Could you check a few things on this model? Use its own coordinates, in mm. A direction names the side the tool comes from. Give positions to 0.01 mm unless a question says otherwise; leave off trailing zeros. Order: outer loops, then holes, each group sorted by start corner. A loop starts at its lowest first (then second) coordinate and runs counter-clockwise, first axis right, second up. Notation, with made-up numbers: M 26,9.5 L 76,9.5 A20 ccw 76,40.5 Z; hole C 39,33 d11. An arc over 180 degrees is marked long. Use a Markdown table: item, result. Add a question column.
```python
from build123d import *

# Parameters (mm, degrees)
BOSS_EXTRU_1_DEPTH = 3


with BuildPart() as part:
    # Esquisse1 → Boss.-Extru.1 (new body)
    with BuildSketch(Plane.XY):
        with BuildLine():
            Line((-119.34630187, 4.320852512), (-119.346382005, -12.429484403))
            Line((-119.346382005, -12.429484403), (-101.345774335, -12.429484403))
            Line((-101.345774335, -12.429484403), (-101.345774335, -9.929307079))
            Line((-101.345774335, -9.929307079), (-82.803225752, -9.929307079))
            Line((-82.803225752, -9.929307079), (-82.803225752, -7.679926158))
            Line((-82.803225752, -7.679926158), (-62.801949021, -7.681038584))
            Line((-62.801949021, -7.681038584), (-62.801949021, -9.929307079))
            Line((-62.801949021, -9.929307079), (-43.80060136, -9.929307079))
            Line((-43.80060136, -9.929307079), (-43.80060136, -14.679643994))
            Line((-43.80060136, -14.679643994), (-5.797906039, -14.679643994))
            Line((-5.797906039, -14.679643994), (-5.797906039, -72.933633781))
            Line((-5.797906039, -72.933633781), (-61.577157206, -72.933633781))
            Line((-61.577157206, -72.933633781), (-72.263087593, -87.572177036))
            Line((-72.263087593, -87.572177036), (-109.761976756, -93.1463556))
            Line((-109.761976756, -93.1463556), (-126.111124489, -102.556497988))
            Line((-126.111124489, -102.556497988), (-140.02282508, -78.342807898))
            Line((-140.02282508, -78.342807898), (-140.02282508, 4.320852512))
            Line((-140.02282508, 4.320852512), (-142.02282508, 4.320852512))
            Line((-142.02282508, 4.320852512), (-154.65055875, 4.320852512))
            Line((-154.65055875, 4.320852512), (-158.478985875, 0.492425388))
            Line((-158.478985875, 0.492425388), (-158.478985875, -3.429484403))
            Line((-158.478985875, -3.429484403), (-158.478985875, -70.307502815))
            Line((-158.478985875, -70.307502815), (-132.440036759, -115.628996046))
            Line((-132.440036759, -115.628996046), (-127.216265437, -117.03834868))
            Line((-127.216265437, -117.03834868), (-105.747438988, -104.681452952))
            Line((-105.747438988, -104.681452952), (-65.531582138, -98.70339941))
            Line((-65.531582138, -98.70339941), (-55.479847181, -84.933633781))
            Line((-55.479847181, -84.933633781), (2.202093961, -84.933633781))
            Line((2.202093961, -84.933633781), (7.202093961, -79.933633781))
            Line((7.202093961, -79.933633781), (7.202093961, -0.684932032))
            Line((7.202093961, -0.684932032), (2.202093969, 4.315346056))
            Line((2.202093969, 4.315346056), (-5.797906039, 4.315790998))
            Line((-5.797906039, 4.315790998), (-5.797906039, -5.684153384))
            ThreePointArc((-5.797906039, -5.684153384), (-6.797906039, -6.684153384), (-7.797906039, -5.684153384))
            Line((-7.797906039, -5.684153384), (-7.797906039, 4.315902234))
            Line((-7.797906039, 4.315902234), (-9.797906039, 4.316013469))
            Line((-9.797906039, 4.316013469), (-9.797906039, -5.684153384))
            ThreePointArc((-9.797906039, -5.684153384), (-10.797906039, -6.684153384), (-11.797906039, -5.684153384))
            Line((-11.797906039, -5.684153384), (-11.797906039, 4.316124705))
            Line((-11.797906039, 4.316124705), (-13.797906039, 4.31623594))
            Line((-13.797906039, 4.31623594), (-13.797906039, -5.684153384))
            ThreePointArc((-13.797906039, -5.684153384), (-14.797906039, -6.684153384), (-15.797906039, -5.684153384))
            Line((-15.797906039, -5.684153384), (-15.797906039, 4.316347176))
            Line((-15.797906039, 4.316347176), (-17.797906039, 4.316458411))
            Line((-17.797906039, 4.316458411), (-17.797906039, -5.684153384))
            ThreePointArc((-17.797906039, -5.684153384), (-18.797906039, -6.684153384), (-19.797906039, -5.684153384))
            Line((-19.797906039, -5.684153384), (-19.797906039, 4.316569647))
            Line((-19.797906039, 4.316569647), (-21.797906039, 4.316680882))
            Line((-21.797906039, 4.316680882), (-21.797906039, -5.684153384))
            ThreePointArc((-21.797906039, -5.684153384), (-22.797906039, -6.684153384), (-23.797906039, -5.684153384))
            Line((-23.797906039, -5.684153384), (-23.797906039, 4.316792118))
            Line((-23.797906039, 4.316792118), (-25.797906039, 4.316903353))
            Line((-25.797906039, 4.316903353), (-25.797906039, -5.684153384))
            ThreePointArc((-25.797906039, -5.684153384), (-26.797906039, -6.684153384), (-27.797906039, -5.684153384))
            Line((-27.797906039, -5.684153384), (-27.797906039, 4.317014589))
            Line((-27.797906039, 4.317014589), (-29.797906039, 4.317125824))
            Line((-29.797906039, 4.317125824), (-29.797906039, -5.684153384))
            ThreePointArc((-29.797906039, -5.684153384), (-30.797906039, -6.684153384), (-31.797906039, -5.684153384))
            Line((-31.797906039, -5.684153384), (-31.797906039, 4.31723706))
            Line((-31.797906039, 4.31723706), (-33.797906039, 4.317348295))
            Line((-33.797906039, 4.317348295), (-33.797906039, -5.684153384))
            ThreePointArc((-33.797906039, -5.684153384), (-34.797906039, -6.684153384), (-35.797906039, -5.684153384))
            Line((-35.797906039, -5.684153384), (-35.797906039, 4.317459531))
            Line((-35.797906039, 4.317459531), (-37.797906039, 4.317570766))
            Line((-37.797906039, 4.317570766), (-37.797906039, -5.684153384))
            ThreePointArc((-37.797906039, -5.684153384), (-38.797906039, -6.684153384), (-39.797906039, -5.684153384))
            Line((-39.797906039, -5.684153384), (-39.797906039, 4.317682002))
            Line((-39.797906039, 4.317682002), (-41.797906039, 4.317793237))
            Line((-41.797906039, 4.317793237), (-41.797906039, -5.684153384))
            ThreePointArc((-41.797906039, -5.684153384), (-42.797906039, -6.684153384), (-43.797906039, -5.684153384))
            Line((-43.797906039, -5.684153384), (-43.797906039, 4.317904473))
            Line((-43.797906039, 4.317904473), (-45.797906039, 4.318015708))
            Line((-45.797906039, 4.318015708), (-45.797906039, -5.684153384))
            ThreePointArc((-45.797906039, -5.684153384), (-46.797906039, -6.684153384), (-47.797906039, -5.684153384))
            Line((-47.797906039, -5.684153384), (-47.797906039, 4.318126944))
            Line((-47.797906039, 4.318126944), (-49.797906039, 4.318238179))
            Line((-49.797906039, 4.318238179), (-49.797906039, -5.684153384))
            ThreePointArc((-49.797906039, -5.684153384), (-50.797906039, -6.684153384), (-51.797906039, -5.684153384))
            Line((-51.797906039, -5.684153384), (-51.797906039, 4.318349415))
            Line((-51.797906039, 4.318349415), (-53.797906039, 4.31846065))
            Line((-53.797906039, 4.31846065), (-53.797906039, -5.684153384))
            ThreePointArc((-53.797906039, -5.684153384), (-54.797906039, -6.684153384), (-55.797906039, -5.684153384))
            Line((-55.797906039, -5.684153384), (-55.797906039, 4.318571886))
            Line((-55.797906039, 4.318571886), (-57.797906039, 4.318683121))
            Line((-57.797906039, 4.318683121), (-57.797906039, -5.684153384))
            ThreePointArc((-57.797906039, -5.684153384), (-58.797906039, -6.684153384), (-59.797906039, -5.684153384))
            Line((-59.797906039, -5.684153384), (-59.797906039, 4.318794357))
            Line((-59.797906039, 4.318794357), (-61.797906039, 4.318905592))
            Line((-61.797906039, 4.318905592), (-61.797906039, -5.684153384))
            ThreePointArc((-61.797906039, -5.684153384), (-62.797906039, -6.684153384), (-63.797906039, -5.684153384))
            Line((-63.797906039, -5.684153384), (-63.797906039, 4.319016828))
            Line((-63.797906039, 4.319016828), (-65.797906039, 4.319128063))
            Line((-65.797906039, 4.319128063), (-65.797906039, -5.684153384))
            ThreePointArc((-65.797906039, -5.684153384), (-66.797906039, -6.684153384), (-67.797906039, -5.684153384))
            Line((-67.797906039, -5.684153384), (-67.797906039, 4.319239299))
            Line((-67.797906039, 4.319239299), (-69.797906039, 4.319350534))
            Line((-69.797906039, 4.319350534), (-69.797906039, -5.684153384))
            ThreePointArc((-69.797906039, -5.684153384), (-70.797906039, -6.684153384), (-71.797906039, -5.684153384))
            Line((-71.797906039, -5.684153384), (-71.797906039, 4.31946177))
            Line((-71.797906039, 4.31946177), (-73.797906039, 4.319573005))
            Line((-73.797906039, 4.319573005), (-73.797906039, -5.684153384))
            ThreePointArc((-73.797906039, -5.684153384), (-74.797906039, -6.684153384), (-75.797906039, -5.684153384))
            Line((-75.797906039, -5.684153384), (-75.797906039, 4.319684241))
            Line((-75.797906039, 4.319684241), (-77.797906039, 4.319795476))
            Line((-77.797906039, 4.319795476), (-77.797906039, -5.684153384))
            ThreePointArc((-77.797906039, -5.684153384), (-78.797906039, -6.684153384), (-79.797906039, -5.684153384))
            Line((-79.797906039, -5.684153384), (-79.797906039, 4.319906712))
            Line((-79.797906039, 4.319906712), (-81.797906039, 4.320017947))
            Line((-81.797906039, 4.320017947), (-81.797906039, -5.684153384))
            ThreePointArc((-81.797906039, -5.684153384), (-82.797906039, -6.684153384), (-83.797906039, -5.684153384))
            Line((-83.797906039, -5.684153384), (-83.797906039, 4.320129183))
            Line((-83.797906039, 4.320129183), (-85.797906039, 4.320240418))
            Line((-85.797906039, 4.320240418), (-85.797906039, -5.684153384))
            ThreePointArc((-85.797906039, -5.684153384), (-86.797906039, -6.684153384), (-87.797906039, -5.684153384))
            Line((-87.797906039, -5.684153384), (-87.797906039, 4.320351654))
            Line((-87.797906039, 4.320351654), (-89.797906039, 4.320462889))
            Line((-89.797906039, 4.320462889), (-89.797906039, -5.684153384))
            ThreePointArc((-89.797906039, -5.684153384), (-90.797906039, -6.684153384), (-91.797906039, -5.684153384))
            Line((-91.797906039, -5.684153384), (-91.797906039, 4.320574125))
            Line((-91.797906039, 4.320574125), (-93.797906039, 4.32068536))
            Line((-93.797906039, 4.32068536), (-93.797906039, -5.684153384))
            ThreePointArc((-93.797906039, -5.684153384), (-94.797906039, -6.684153384), (-95.797906039, -5.684153384))
            Line((-95.797906039, -5.684153384), (-95.797906039, 4.320796596))
            Line((-95.797906039, 4.320796596), (-96.80328137, 4.320852512))
            Line((-96.80328137, 4.320852512), (-97.797906039, 4.320852512))
            Line((-97.797906039, 4.320852512), (-97.797906039, -5.684153384))
            ThreePointArc((-97.797906039, -5.684153384), (-98.797906039, -6.684153384), (-99.797906039, -5.684153384))
            Line((-99.797906039, -5.684153384), (-99.797906039, 4.320852512))
            Line((-99.797906039, 4.320852512), (-101.797906039, 4.320852512))
            Line((-101.797906039, 4.320852512), (-101.797906039, -5.684153384))
            ThreePointArc((-101.797906039, -5.684153384), (-102.797906039, -6.684153384), (-103.797906039, -5.684153384))
            Line((-103.797906039, -5.684153384), (-103.797906039, 4.320852512))
            Line((-103.797906039, 4.320852512), (-103.799739609, 4.320852512))
            Line((-103.799739609, 4.320852512), (-117.346315028, 4.320852512))
            Line((-117.346315028, 4.320852512), (-119.34630187, 4.320852512))
        make_face()
    extrude(amount=BOSS_EXTRU_1_DEPTH)


solid = part.part
```
1) Suppose I cut it at B-B on y = -95.5. Please give me the cut outline in (x, z), and give its area (3 significant figures).
2) For faces 1 (the face through (-51, -74, 3)), 2 (the face through (-66.845, -80.15, 1.479)), 3 (the face through (-132.97, -90.62, 1.48)), which set-ups out of +Z, -Z, +X, -X, +Y, -Y let a thin tool reach every point of the face, with its end or its side?
3) Please list where these lines run through material, in increasing order: line 1 (X direction, y = -10.5, z = 1); line 2 (Y direction, x = -59, z = 2.35); line 3 (X direction, y = -69.5, z = 0.65). Write a range as from..to.
4) For pin 1 (0.9 mm diameter, centred on y = 1, z = 1.5, fed in from -X); pin 2 (1.5 mm diameter, centred on y = 0.5, z = 2, fed in from +X); pin 3 (1 mm diameter, centred on x = -48.5, z = 1, fed in from +Y), each with a flat end and sliding along its axis, tell me the tip position at first contact or that it passes through.
5) Suppose I cut it at C-C on x = -129. Please give me the cut outline in (y, z), and give its area (3 significant figures).
6) Suppose I cut it at A-A on y = -56. Please give me the cut outline in (x, z), and give its area (3 significant figures).
7) We'd pull the mould along X, two halves only. Please class faces 4 (the face through (-90.75, -90.32, 1.48)), 5 (the face through (-145.642, -92.651, 1.479)), 6 (the face through (-60.576, -91.915, 1.479)), 7 (the face through (-117.822, -97.786, 1.479)): pulls with the +X half, pulls with the -X half, needs draft (parallel to the pull), parting line crosses it, or undercut.
Values found:
| question | item | result |
|---|---|---|
| 1 | outline | M -144,0 L -130.17,0 L -130.17,3 L -144,3 Z; M -113.85,0 L -63.19,0 L -63.19,3 L -113.85,3 Z |
| 1 | area | 193 mm^2 |
| 2 | face 1 | +Z, +X, -X, +Y, -Y |
| 2 | face 2 | +Z, -Z |
| 2 | face 3 | +Z, -Z, +Y |
| 3 | line 1 | x = -158.48..-140.02, -119.35..-101.35, -43.8..7.2 |
| 3 | line 2 | y = -89.76..-72.93, -9.93..-6.66 |
| 3 | line 3 | x = -158.48..-140.02, -5.8..7.2 |
| 4 | pin 1 | stops at x = -158.42 |
| 4 | pin 2 | stops at x = 6.77 |
| 4 | pin 3 | stops at y = 4.32 |
| 5 | outline | M -116.56,0 L -97.53,0 L -97.53,3 L -116.56,3 Z |
| 5 | area | 57.1 mm^2 |
| 6 | outline | M -158.48,0 L -140.02,0 L -140.02,3 L -158.48,3 Z; M -5.8,0 L 7.2,0 L 7.2,3 L -5.8,3 Z |
| 6 | area | 94.4 mm^2 |
| 7 | face 4 | undercut |
| 7 | face 5 | pulls with the -X half |
| 7 | face 6 | pulls with the +X half |
| 7 | face 7 | undercut |
